Source: CAD feature listing. Evaluate the final solid. Frame: model axes, mm. A direction names the side the tool comes from. Round coordinates to 2 decimals unless told otherwise and drop trailing zeros. Loops run counter-clockwise (first coordinate to the right, second up) from the corner with the lowest first, then second, coordinate; pieces in that order, holes last.
(1) Section C-C, the plane x = 5.4. Return the cut outline in (y, z).
(2) First-contact query: pin 1 Ø3 at (y, z) = (-3.5, -5) entering from -X (3 decimals); pin 2 Ø1.5 at (x, y) = (-1, 6.5) entering from -Z; pin 3 Ø0.5 at (x, z) = (-6.5, -5.5) entering from +Y. Flat tips, straight axial feed; report the tip coordinate or a pass-through.
(3) Mould query, pull axis Y, two halves, no side actions, for faces 3 (the flat face through (8.05, 0, 1)), 4 (the flat face through (-1.7, 10.25, 0.4)), 5 (the flat face through (-7, 0, -3)). Classes: pulls with the +Y half, pulls with the -Y half, needs draft (parallel to the pull), parting line crosses it, or undercut.
(4) Section B-B, the plane y = 7.35. Return the cut outline in (x, z).
(5) Set-up query: faces 1 (the flat face through (0, 0, 1.63)), 2 (the flat face through (1, 0, 0)). Return all of +Z, -Z, +X, -X, +Y, -Y with unobstructed straight access to the full face (end or side cutting, diameter ignored); none if empty.
(6) Section D-D, the plane z = 0.5. Return the cut outline in (x, y).
(7) Material intervals for probe 1 along Y at (x, z) = (5.4, 0.9); probe 2 along Z at (x, y) = (-5, -2.25); probe 3 along X at (y, z) = (6, -2.5), sorted ascending.
(8) Section A-A, the plane z = -6.25. Count the separate pieces of the cut face and the enclosed holes in it, plus the area to 3 significant figures.
```python
from build123d import *

# Parameters (mm, degrees)
SKETCH1_W               = 16.1
SKETCH1_H               = 20.5
BOSS_EXTRUDE1_DEPTH     = 1.63
CUT_EXTRUDE1_DEPTH      = 14.134759229
CUT_EXTRUDE1_DEPTH_BACK = 14.134759229
SKETCH2_R               = 1.65
SKETCH3_W               = 2.6
SKETCH3_H               = 20.5
BOSS_EXTRUDE2_DEPTH     = 3
SKETCH4_W               = 0.63
SKETCH4_H               = 0.63
BOSS_EXTRUDE3_DEPTH     = 4.37


with BuildPart() as part:
    # Sketch1 → Boss-Extrude1 (new body)
    with BuildSketch(Plane.XY):
        Rectangle(SKETCH1_W, SKETCH1_H)
    extrude(amount=BOSS_EXTRUDE1_DEPTH)

    # Sketch2 → Cut-Extrude1 (cut, two sides: drawn at the far end of the back side and taken through both)
    with BuildSketch(Plane.XY.offset(1.63).offset(-CUT_EXTRUDE1_DEPTH_BACK)):
        with Locations((5.4, 7.35)):
            Circle(SKETCH2_R)
        with Locations((5.4, -7.35)):
            Circle(SKETCH2_R)
    extrude(amount=CUT_EXTRUDE1_DEPTH + CUT_EXTRUDE1_DEPTH_BACK, mode=Mode.SUBTRACT)

    # Sketch3 → Boss-Extrude2 (add)
    with BuildSketch(Plane(origin=(0, 0, 0), x_dir=(-1, 0, 0), z_dir=(0, 0, -1))):
        with Locations((6.75, 0)):
            Rectangle(SKETCH3_W, SKETCH3_H)
    extrude(amount=BOSS_EXTRUDE2_DEPTH)

    # Sketch4 → Boss-Extrude3 (add)
    with BuildSketch(Plane(origin=(0, 0, -3), x_dir=(-1, 0, 0), z_dir=(0, 0, -1))):
        with Locations((6.75, 8.855)):
            Rectangle(SKETCH4_W, SKETCH4_H)
        with Locations((6.75, 6.325)):
            Rectangle(SKETCH4_W, SKETCH4_H)
        with Locations((6.75, 3.795)):
            Rectangle(SKETCH4_W, SKETCH4_H)
        with Locations((6.75, 1.265)):
            Rectangle(SKETCH4_W, SKETCH4_H)
        with Locations((6.75, -1.265)):
            Rectangle(SKETCH4_W, SKETCH4_H)
        with Locations((6.75, -3.795)):
            Rectangle(SKETCH4_W, SKETCH4_H)
        with Locations((6.75, -6.325)):
            Rectangle(SKETCH4_W, SKETCH4_H)
        with Locations((6.75, -8.855)):
            Rectangle(SKETCH4_W, SKETCH4_H)
    extrude(amount=BOSS_EXTRUDE3_DEPTH)


solid = part.part
```
Output values:
1. outline: (-10.25, 0) - (-9, 0) - (-9, 1.63) - (-10.25, 1.63) - close; (-5.7, 0) - (5.7, 0) - (5.7, 1.63) - (-5.7, 1.63) - close; (9, 0) - (10.25, 0) - (10.25, 1.63) - (9, 1.63) - close
2. pin 1: stops at x = -7.065
2. pin 2: stops at z = 0
2. pin 3: stops at y = 9.17
3. face 3: needs draft
3. face 4: pulls with the +Y half
3. face 5: undercut
4. outline: (-8.05, -3) - (-5.45, -3) - (-5.45, 0) - (3.75, 0) - (3.75, 1.63) - (-8.05, 1.63) - close; (7.05, 0) - (8.05, 0) - (8.05, 1.63) - (7.05, 1.63) - close
5. face 1: +Z, +X, -X, +Y, -Y
5. face 2: -Z, +X, +Y, -Y
6. outline: (-8.05, -10.25) - (8.05, -10.25) - (8.05, 10.25) - (-8.05, 10.25) - close; hole circle Ø3.3 at (5.4, -7.35); hole circle Ø3.3 at (5.4, 7.35)
7. probe 1: y = -10.25 to -9, -5.7 to 5.7, 9 to 10.25
7. probe 2: z = 0 to 1.63
7. probe 3: x = -8.05 to -5.45
8. separate pieces: 8
8. enclosed holes: 0
8. area: 3.18 mm2
